Could you check a few things on this drawing? It's one solid part, dimensions in mm from its lowest x, y, z. A direction names the side the tool comes from. Coordinates: 2 decimals unless noted, no trailing zeros. Loops run counter-clockwise (first coordinate to the right, second up) from the corner with the lowest first, then second, coordinate; pieces in that order, holes last.
1) Will these pins go through, and if not, where does the flat tip stop? P1, Ø4, axis at x = 47, z = 12, coming from the -Y side; P2, Ø4, axis at x = 34.5, y = 3.5, coming from the +Z side; P3, Ø8, axis at x = 51, y = 15, coming from the +Z side.
2) Imagine slicing it at C-C on x = 5. Please give me the cut outline in (y, z), plus the area to 3 significant figures.
3) Imagine slicing it at A-A on z = 22.5. Please give me the cut outline in (x, y).
4) For the marked faces 1 and 2, which set-ups out of +Z, -Z, +X, -X, +Y, -Y let a thin tool reach every point of the face, with its end or its side?
5) Imagine slicing it at B-B on y = 14.5. Please give me the cut outline in (x, z), plus the area to 3 significant figures.
6) Imagine slicing it at D-D on x = 50. Please give me the cut outline in (y, z).
7) If I drill on line 1 along Z through (x, y) = (20.5, 4.75); line 2 along X through (y, z) = (8.25, 8.25); line 3 along X through (y, z) = (7.5, 18), over which ranges is the centre line in solid material (lowest first)?
8) Thinking about a two-plate mould opening in X: for the marked faces 3, 4 and 5, which applies, released by +X, released by -X, zero draft, split by the parting line, or undercut?
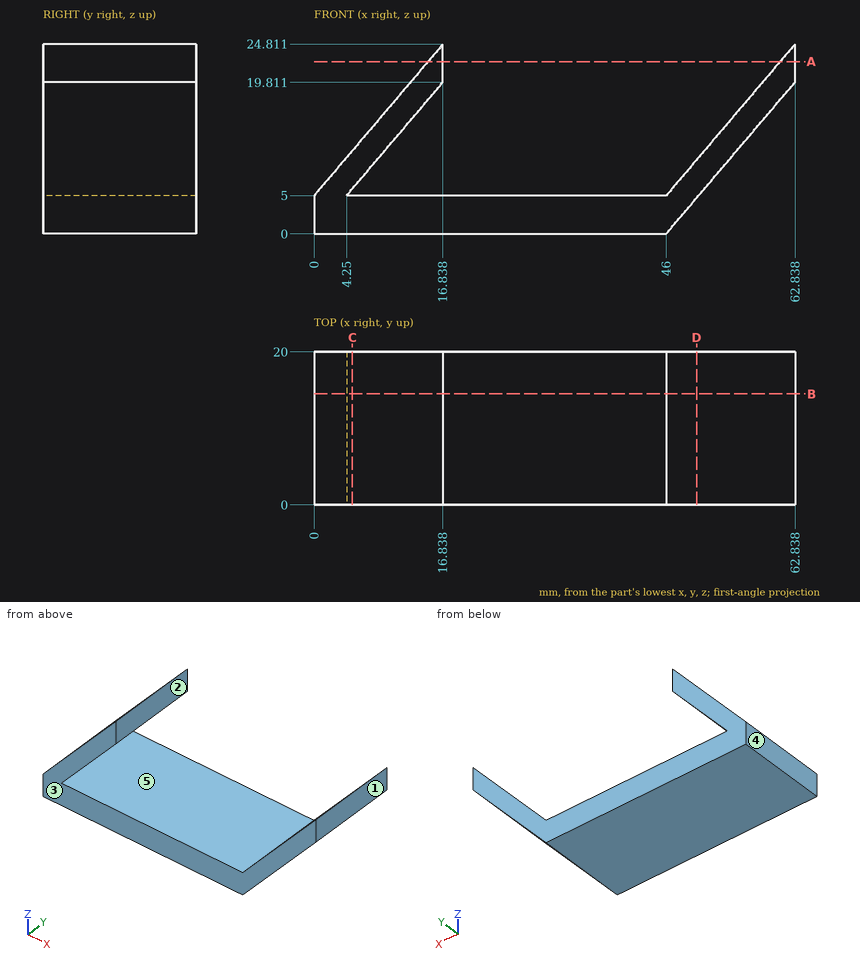
Filled in:
1. P1: passes through
1. P2: stops at z = 5
1. P3: stops at z = 15.59
2. outline: (0, 0) - (20, 0) - (20, 5) - (0, 5) - close; (0, 5.88) - (20, 5.88) - (20, 10.88) - (0, 10.88) - close
2. area: 200 mm2
3. outline: (14.87, 0) - (16.84, 0) - (16.84, 20) - (14.87, 20) - close; (60.87, 0) - (62.84, 0) - (62.84, 20) - (60.87, 20) - close
4. face 1: +Z, -Z, +X, +Y, -Y
4. face 2: +Z, +Y, -Y
5. outline: (0, 0) - (46, 0) - (62.84, 19.81) - (62.84, 24.81) - (46, 5) - (4.25, 5) - (16.84, 19.81) - (16.84, 24.81) - (0, 5) - close
5. area: 388 mm2
6. outline: (0, 4.71) - (20, 4.71) - (20, 9.71) - (0, 9.71) - close
7. line 1: z = 0 to 5
7. line 2: x = 2.76 to 7.01, 48.76 to 53.01
7. line 3: x = 11.05 to 15.3, 57.05 to 61.3
8. face 3: zero draft
8. face 4: released by -X
8. face 5: undercut
